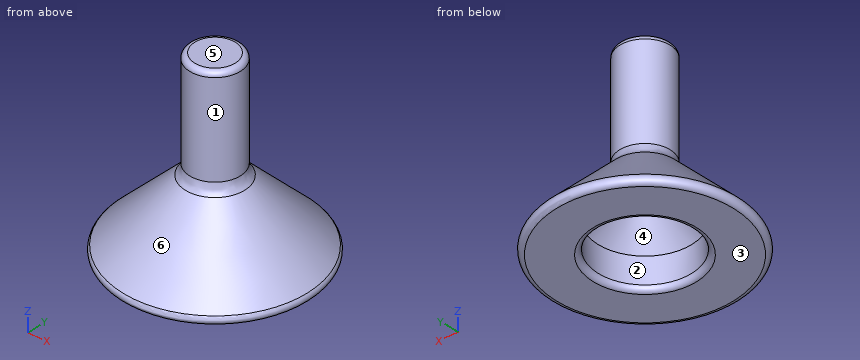
from build123d import *

# Parameters (mm, degrees)
FILLET001_R = 6
FILLET003_R = 2


with BuildPart() as part:
    # Sketch → Revolution (revolve)
    with BuildSketch(Plane.XZ):
        Polygon((18.55, 0), (18.55, 12.2), (6.05, 24.7), (0, 24.7), (0, 71.45), (10, 71.45), (10, 30), (40, 0), align=None)
    revolve(axis=Axis((0, 0, 0), (0, 0, 1)))

    # Fillet001
    fillet001_edges = [part.edges().sort_by_distance(p)[0] for p in [
        (-10, 0, 30),
    ]]
    fillet(fillet001_edges, radius=FILLET001_R)

    # Fillet003
    fillet003_edges = [part.edges().sort_by_distance(p)[0] for p in [
        (-10, 0, 71.45),
        (-18.55, 0, 0),
        (-40, 0, 0),
    ]]
    fillet(fillet003_edges, radius=FILLET003_R)


solid = part.part
Geometry: final body of the model. Coordinates: model frame, mm. Face numbers are marked on the shaded views. A direction names the side the tool comes from. Coordinates: 2 decimals unless noted, no trailing zeros. Order: outer loops, then holes, each group sorted by start corner. A loop starts at its lowest first (then second) coordinate and runs counter-clockwise, first axis right, second up. Notation, with made-up numbers: M 6,86 L 10,86 A9 ccw 10,92 Z; hole C 47,55 d10. An arc over 180 degrees is marked long. One line per question, with ' | ' between items. Start each with the question number.
Item 1: Ray query, probe 1 along Y at (x, z) = (0, 10); probe 2 along Y at (x, z) = (5, 5.5); probe 3 along Z at (x, y) = (4.5, -17.5). Return the intervals inside material, ascending. Write a range as [from, to].
Item 2: Draft query along Y for the marked faces 4, 5 and 6. Return one class per face: released by +Y, released by -Y, zero draft, split by the parting line, or undercut.
Item 3: Pin query (flat end, axial travel): pin 1 Ø12 at (x, y) = (20.5, -7.5) entering from +Z; pin 2 Ø5 at (y, z) = (-23.5, 10) entering from +X; pin 3 Ø3 at (y, z) = (-10.5, 46) entering from -X. Return the tip coordinate at first contact, or that it passes through.
Item 4: Cut plane C-C, the plane z = 6. Return the cut outline in (x, y), then the cut area to 3 significant figures.
Item 5: Cut plane A-A, the plane z = 23. Return the cut outline in (x, y).
Item 6: Set-up query: the marked faces 1, 2 and 3. Return all of +Z, -Z, +X, -X, +Y, -Y with unobstructed straight access to the full face (end or side cutting, diameter ignored); none if empty.
Item 7: Cut plane B-B, the plane z = 38.5. Return the cut outline in (x, y), then the cut area to 3 significant figures.
A:
1) probe 1: y = [-30, -18.55], [18.55, 30] | probe 2: y = [-34.14, -17.86], [17.86, 34.14] | probe 3: z = [12.68, 21.93]
2) face 4: undercut | face 5: zero draft | face 6: split by the parting line
3) pin 1: stops at z = 24.17 | pin 2: stops at x = 23.24 | pin 3: stops at x = -4.36
4) outline: C 0,0 d68; hole C 0,0 d37.1 | area: 2,550 mm2
5) outline: C 0,0 d34; hole C 0,0 d15.5
6) face 1: +Z | face 2: -Z | face 3: -Z, +X, -X, +Y, -Y
7) outline: C 0,0 d20 | area: 314 mm2
